from build123d import *

# Parameters (mm, degrees)
SKETCH2_R               = 2.025
SKETCH2_R_2             = 5
BOSS_EXTRUDE3_DEPTH     = 2
BOSS_EXTRUDE4_START     = -50
BOSS_EXTRUDE4_DEPTH     = 52
BOSS_EXTRUDE6_START     = -30
SKETCH7_W               = 37.7
SKETCH7_H               = 28.7
SKETCH7_R               = 9.4
BOSS_EXTRUDE6_DEPTH     = 30
BOSS_EXTRUDE7_START     = -26.7
BOSS_EXTRUDE7_DEPTH     = 26.7
CUT_EXTRUDE1_DEPTH      = 82.633709336
CUT_EXTRUDE1_DEPTH_BACK = 82.633709336
SKETCH6_R               = 3.975
RIB3_START              = -5
RIB3_DEPTH              = 10
FILLET2_R               = 4


# Read off the part's stored shape, not the designer's step: Rib3
with BuildPart() as part:
    # Sketch2 → Boss-Extrude3 (new body)
    with BuildSketch(Plane.XY):
        with BuildLine():
            Line((12.5, -30), (12.5, -13.297086147))
            ThreePointArc((12.5, -13.297086147), (0, 18.25), (-12.5, -13.297086147))
            Line((-12.5, -13.297086147), (-12.5, -30))
            Line((-12.5, -30), (12.5, -30))
        make_face()
        with Locations((8, 8)):
            Circle(SKETCH2_R, mode=Mode.SUBTRACT)
        with Locations((-8, -8)):
            Circle(SKETCH2_R, mode=Mode.SUBTRACT)
        with Locations((-8, 8)):
            Circle(SKETCH2_R, mode=Mode.SUBTRACT)
        with Locations((8, -8)):
            Circle(SKETCH2_R, mode=Mode.SUBTRACT)
        Circle(SKETCH2_R_2, mode=Mode.SUBTRACT)
    extrude(amount=BOSS_EXTRUDE3_DEPTH)

    # Sketch3 → Boss-Extrude4 (add)
    with BuildSketch(Plane.XY.offset(BOSS_EXTRUDE4_START)):
        with BuildLine():
            Line((23.75, 0), (18.25, 0))
            ThreePointArc((18.25, 0), (0, -18.25), (-18.25, 0))
            Line((-18.25, 0), (-23.75, 0))
            ThreePointArc((-23.75, 0), (0, -23.75), (23.75, 0))
        make_face()
    extrude(amount=BOSS_EXTRUDE4_DEPTH)

    # Sketch7 → Boss-Extrude6 (add)
    with BuildSketch(Plane(origin=(0, 0, 0), x_dir=(1, 0, 0), z_dir=(0, 1, 0)).offset(BOSS_EXTRUDE6_START)):
        with Locations((0, 12.35)):
            Rectangle(SKETCH7_W, SKETCH7_H)
        with Locations(Location((0, 12.35, 0), (0, 0, 180))):
            Circle(SKETCH7_R, mode=Mode.SUBTRACT)
    extrude(amount=-BOSS_EXTRUDE6_DEPTH)

    # Sketch2<8> → Boss-Extrude7 (add)
    with BuildSketch(Plane.XY.offset(BOSS_EXTRUDE7_START)):
        with BuildLine():
            Line((12.5, -30), (12.5, -13.297086147))
            ThreePointArc((12.5, -13.297086147), (0, -18.25), (-12.5, -13.297086147))
            Line((-12.5, -13.297086147), (-12.5, -30))
            Line((-12.5, -30), (12.5, -30))
        make_face()
    extrude(amount=BOSS_EXTRUDE7_DEPTH)

    # Sketch6 → Cut-Extrude1 (cut, two sides: drawn at the far end of the back side and taken through both)
    with BuildSketch(Plane(origin=(0, 0, 0), x_dir=(0, 0, -1), z_dir=(1, 0, 0)).offset(-CUT_EXTRUDE1_DEPTH_BACK)):
        with Locations((12.35, -40)):
            Circle(SKETCH6_R)
        with Locations((12.35, -52.5)):
            Circle(SKETCH6_R)
    extrude(amount=CUT_EXTRUDE1_DEPTH + CUT_EXTRUDE1_DEPTH_BACK, mode=Mode.SUBTRACT)

    # Rib3 outline → Rib3 (add)
    with BuildSketch(Plane(origin=(0, -60, 0), x_dir=(0, -1, 0), z_dir=(-1, 0, 0)).offset(RIB3_START)):
        Polygon((-38, -50), (-31.25, -50), (0, -26.7), (-38, -26.7), align=None)
    extrude(amount=RIB3_DEPTH)

    # Fillet2
    fillet2_edges = [part.edges().sort_by_distance(p)[0] for p in [
        (12.5, -30, -12.35),
        (-12.5, -30, -12.35),
        (-18.25, 0, 1),
        (12.5, -20.194368027, -12.35),
        (18.25, 0, 1),
        (-12.5, -20.194368027, -12.35),
    ]]
    fillet(fillet2_edges, radius=FILLET2_R)


solid = part.part
Input: part model. Units: mm. Frame: model coordinates. A direction names the side the tool comes from. Give positions to 0.01 mm unless a question says otherwise; leave off trailing zeros. Write each loop counter-clockwise with the first axis right and the second up, starting at its lowest first coordinate (ties: lowest second). Pieces come first, ordered by that corner, then holes. Notation, with made-up numbers: (42, 79.5) -> (72, 79.5) arc R32 cw to (72, 109.5) -> close; hole circle Ø3 at (45.5, 4.5). An arc over 180 degrees is marked (long way). Use one line per item in the form item = value. Start each with the question number.
1) Section query A-A on x = 0. Return the cut outline in (y, z).
2) Section query B-B on y = -50.5. Return the cut outline in (x, z), then the cut area to 3 significant figures.
3) Section query D-D on x = -7. Return the cut outline in (y, z), then the cut area to 3 significant figures.
4) Draft query along Y for faces 1 (the flat face through (21, 0, -24)), 2 (the cylindrical face through (-1.08, -4.88, 0.99)), 3 (the flat face through (-5.2, 0.3, 0)). Return one class per face: pulls with the +Y half, pulls with the -Y half, needs draft (parallel to the pull), parting line crosses it, or undercut.
5) Section query C-C on z = -23. Return the cut outline in (x, y).
6) Ray query, probe 1 along Y at (x, z) = (8, 0.55) (3 decimals); probe 2 along Z at (x, y) = (-17, -40) (3 decimals); probe 3 along Y at (x, z) = (-14.75, -12.35) (3 decimals). Return the intervals inside material, ascending. Write a range as from..to.
7) Set-up query: faces 4 (the flat face through (-18, -30, -13)), 5 (the flat face through (12.5, -24, -13)), 6 (the flat face through (-5, -37, -36)), 7 (the flat face through (5, -37, -36)). Return all of +Z, -Z, +X, -X, +Y, -Y with unobstructed straight access to the full face (end or side cutting, diameter ignored); none if empty.
8) Pin query (flat end, axial travel): pin 1 (1.5 mm diameter, centred on x = 14.5, z = -42.5, fed in from -Y); pin 2 (5 mm diameter, centred on x = -11.5, z = -42, fed in from -Y); pin 3 (4.5 mm diameter, centred on x = 8, y = -8, fed in from -Z). Return the tip coordinate at first contact, or that it passes through.
Outcome:
q1.outline = (-60, -26.7) -> (-28.75, -50) -> (-18.25, -50) -> (-18.25, 0) -> (-5, 0) -> (-5, 2) -> (-60, 2) -> (-60, -2.95) -> (-30, -2.95) -> (-30, -21.75) -> (-60, -21.75) -> close; (5, 0) -> (18.25, 0) -> (18.25, 2) -> (5, 2) -> close
q2.outline = (-18.85, -26.7) -> (-5, -26.7) -> (-5, -33.78) -> (5, -33.78) -> (5, -26.7) -> (18.85, -26.7) -> (18.85, -15.79) -> (8.75, -15.79) arc R9.4 cw to (-8.75, -15.79) -> (-18.85, -15.79) -> close; (-18.85, -8.91) -> (-8.75, -8.91) arc R9.4 cw to (8.75, -8.91) -> (18.85, -8.91) -> (18.85, 2) -> (-18.85, 2) -> close
q2.area = 742 mm^2
q3.outline = (-60, -26.7) -> (-22.69, -26.7) -> (-22.69, -50) -> (-16.85, -50) -> (-16.85, 0) -> (-9.76, 0) -> (-9.76, 2) -> (-60, 2) -> (-60, -6.08) -> (-30, -6.08) -> (-30, -18.62) -> (-60, -18.62) -> close; (-6.24, 0) -> (6.24, 0) -> (6.24, 2) -> (-6.24, 2) -> close; (9.76, 0) -> (16.85, 0) -> (16.85, 2) -> (9.76, 2) -> close
q3.area = 1,050 mm^2
q4.face_1 = pulls with the +Y half
q4.face_2 = undercut
q4.face_3 = needs draft
q5.outline = (-23.75, 0) arc R23.75 ccw to (-14.12, -19.1) arc R4 cw to (-12.5, -22.31) -> (-12.5, -26) arc R4 cw to (-16.5, -30) -> (-18.85, -30) -> (-18.85, -60) -> (18.85, -60) -> (18.85, -30) -> (16.5, -30) arc R4 cw to (12.5, -26) -> (12.5, -22.31) arc R4 cw to (14.12, -19.1) arc R23.75 ccw to (23.75, 0) -> (18.25, 0) arc R18.25 cw to (-18.25, 0) -> close
q6.probe_1 = -60..-10.025, -5.975..5.975, 10.025..16.403
q6.probe_2 = -26.7..-16.325, -8.375..2
q6.probe_3 = -60..-56.475, -48.525..-43.975, -36.025..-29.597, -18.615..-10.747
q7.face_4 = +Z, -Z, -X
q7.face_5 = +Z, -Z, +X
q7.face_6 = -Z, -X, -Y
q7.face_7 = -Z, +X, -Y
q8.pin_1 = -19.36
q8.pin_2 = -21.98
q8.pin_3 = 0
